from build123d import *

# Parameters (mm, degrees)
CUT_EXTRUDE_1_DEPTH = 10


with BuildPart() as part:
    # 草图1 → 旋转1 (revolve)
    with BuildSketch(Plane.XY, mode=Mode.PRIVATE) as revolve_1_sk:
        Polygon((0, 0), (0, 20), (18, 20), (18, 19.75), (111, 19.75), (111, 20), (129, 20), (129, 25), (192, 25), (192, 20), (237, 20), (237, 19.75), (277, 19.75), (277, 20), (322, 20), (322, 18), (337, 18), (337, 17.5), (355, 17.5), (355, 0), align=None)
    revolve(revolve_1_sk.sketch.rotate(Axis((0, 0, 0), (-1, 0, 0)), 90), axis=Axis((0, 0, 0), (-1, 0, 0)))

    # 草图2 → 切除-拉伸1 (cut)
    with BuildSketch(Plane.XY.offset(15)):
        with BuildLine():
            Line((200, 6), (230, 6))
            ThreePointArc((230, 6), (236, 0), (230, -6))
            Line((230, -6), (200, -6))
            ThreePointArc((200, -6), (194, 0), (200, 6))
        make_face()
        with BuildLine():
            Line((285, 6), (315, 6))
            ThreePointArc((315, 6), (321, 0), (315, -6))
            Line((315, -6), (285, -6))
            ThreePointArc((285, -6), (279, 0), (285, 6))
        make_face()
    extrude(amount=CUT_EXTRUDE_1_DEPTH, mode=Mode.SUBTRACT)


solid = part.part
Check sheet for the modelled part. Datum: model origin and axes. Units: mm. A direction names the side the tool comes from. Coordinates: 2 decimals unless noted, no trailing zeros. Loops run counter-clockwise (first coordinate to the right, second up) from the corner with the lowest first, then second, coordinate; pieces in that order, holes last. Notation, with made-up numbers: (72.5, -17) -> (120.5, -17) arc R16 ccw to (120.5, -9) -> close; hole circle Ø8 at (-40, 3.25). An arc over 180 degrees is marked (long way). Write item = value, one per line. Start each with the question number.
1. Section check A-A on x = 49.5. Record the cut outline in (y, z).
2. Depth check by flat-ended pin: P1, Ø2, axis at x = 302.5, z = 17, coming from the -Y side; P2, Ø4.5, axis at x = 210.5, z = 17, coming from the -Y side; P3, Ø8, axis at x = 174.5, y = -11, coming from the +Z side. Enter the tip coordinate at first touch or a pass-through.
3. Material ranges on line 1 (X direction, y = 7, z = -21.5); line 2 (Z direction, x = 294.5, y = -3); line 3 (Y direction, x = 266.5, z = 0), recorded low to high.
4. Draft check along Y on faces 1 (the flat face through (355, 0, 0)), 2 (the cylindrical face through (120.13, -0.88, 19.98)), 3 (the flat face through (215, 0, 15)). Enter one of: released by +Y, released by -Y, zero draft, split by the parting line, or undercut.
5. Section check B-B on x = 187. Record the cut outline in (y, z).
6. Tool access check on faces 4 (the flat face through (129, -17, -11)), 5 (the flat face through (0, 0, 0)), 6 (the cylindrical face through (321, 0, 17)), 7 (the cylindrical face through (329.605, -12.165, 13.267)). Record the directions out of +Z, -Z, +X, -X, +Y, -Y that give a thin tool (end or side, any length) a straight path to the whole face; none if there is none.
Responses:
q1.outline = circle Ø39.5 at (0, 0)
q2.P1 = -12
q2.P2 = -13.51
q2.P3 = 24
q3.line_1 = 129 to 192
q3.line_2 = -19.77 to 15
q3.line_3 = -19.75 to 19.75
q4.face_1 = zero draft
q4.face_2 = split by the parting line
q4.face_3 = undercut
q5.outline = circle Ø50 at (0, 0)
q6.face_4 = -X
q6.face_5 = +Z, -Z, -X, +Y, -Y
q6.face_6 = +Z
q6.face_7 = +X
